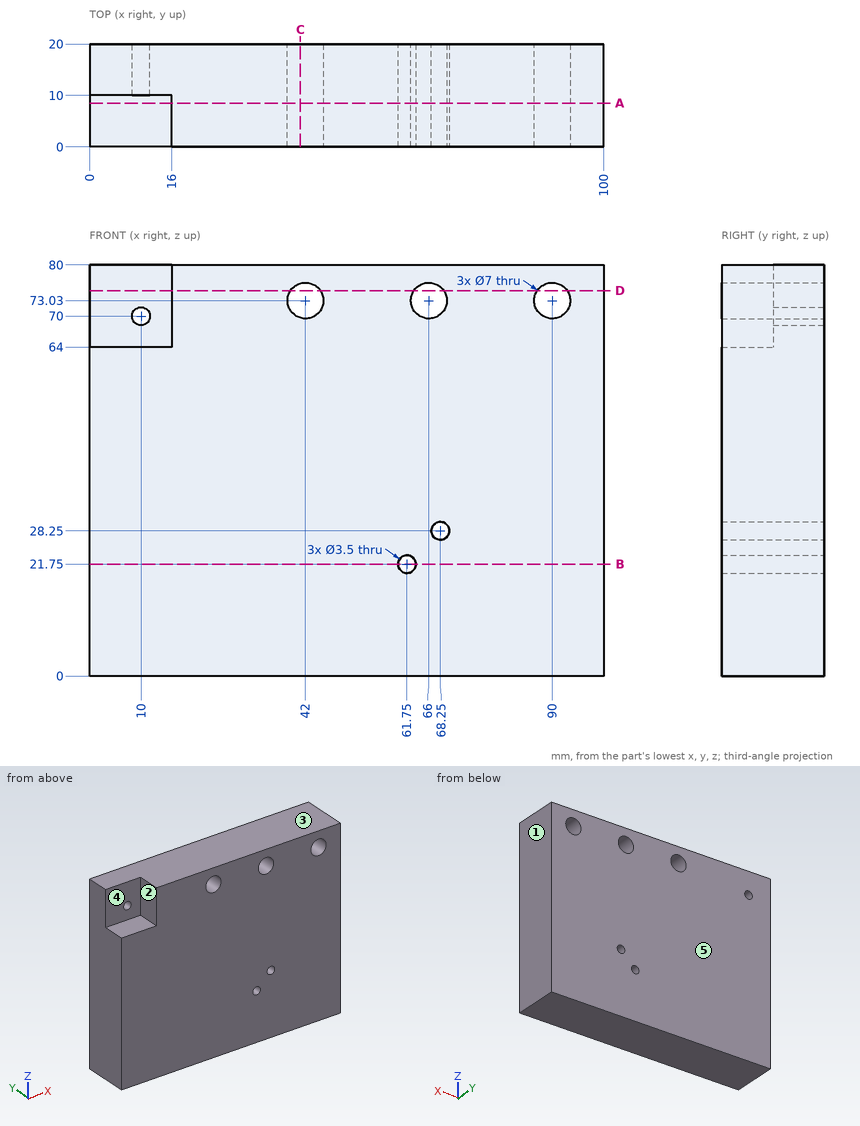
Input: dimensioned drawing with shaded views. Units: mm. Origin: part minimum x, y, z. A direction names the side the tool comes from. Give positions to 0.01 mm unless a question says otherwise; leave off trailing zeros. Order: outer loops, then holes, each group sorted by start corner. A loop starts at its lowest first (then second) coordinate and runs counter-clockwise, first axis right, second up. Notation, with made-up numbers: (70.25, -24.5) -> (117.25, -24.5) arc R14 cw to (117.25, -14.5) -> close; hole circle Ø11 at (85, 43). An arc over 180 degrees is marked (long way). Write item = value, one per line.
Item 1: Ray query, probe 1 along Z at (x, y) = (66, 14); probe 2 along X at (y, z) = (16.5, 70); probe 3 along X at (y, z) = (9.5, 74). Return the intervals inside material, ascending.
Check result:
probe_1 = 0 to 69.53, 76.53 to 80
probe_2 = 0 to 8.25, 11.75 to 40.25, 43.75 to 64.25, 67.75 to 88.25, 91.75 to 100
probe_3 = 16 to 38.64, 45.36 to 62.64, 69.36 to 86.64, 93.36 to 100
Item 2: Contact query for flat-ended pins moving along their axis: pin 1 (4 mm diameter, centred on x = 66, z = 73.03, fed in from -Y); pin 2 (5 mm diameter, centred on x = 9, y = 3, fed in from +Z). Output: stop coordinate, or through.
Check result:
pin_1 = through
pin_2 = 64
Item 3: Section query D-D (z = 75). Output: boundary loops of the cut face in (x, y), then the cut area to 3 significant figures.
Check result:
outline = (0, 10) -> (16, 10) -> (16, 0) -> (39.11, 0) -> (39.11, 20) -> (0, 20) -> close; (44.89, 0) -> (63.11, 0) -> (63.11, 20) -> (44.89, 20) -> close; (68.89, 0) -> (87.11, 0) -> (87.11, 20) -> (68.89, 20) -> close; (92.89, 0) -> (100, 0) -> (100, 20) -> (92.89, 20) -> close
area = 1,490 mm²
Item 4: Section query B-B (z = 21.75). Output: boundary loops of the cut face in (x, y), then the cut area to 3 significant figures.
Check result:
outline = (0, 0) -> (60, 0) -> (60, 20) -> (0, 20) -> close; (63.5, 0) -> (100, 0) -> (100, 20) -> (63.5, 20) -> close
area = 1,930 mm²
Item 5: Mould query, pull axis X, two halves, no side actions, for the marked faces 1, 2 and 3. Classes: +X half, -X half, draft (parallel to the pull), parting line (faces both ways), or undercut.
Check result:
face_1 = +X half
face_2 = -X half
face_3 = draft
Item 6: Section query A-A (y = 8.5). Output: boundary loops of the cut face in (x, z), then the cut area to 3 significant figures.
Check result:
outline = (0, 0) -> (100, 0) -> (100, 80) -> (16, 80) -> (16, 64) -> (0, 64) -> close; hole circle Ø7 at (42, 73.03); hole circle Ø3.5 at (61.75, 21.75); hole circle Ø7 at (66, 73.03); hole circle Ø3.5 at (68.25, 28.25); hole circle Ø7 at (90, 73.03)
area = 7,610 mm²
Item 7: Section query C-C (x = 41). Output: boundary loops of the cut face in (y, z).
Check result:
outline = (0, 0) -> (20, 0) -> (20, 69.68) -> (0, 69.68) -> close; (0, 76.38) -> (20, 76.38) -> (20, 80) -> (0, 80) -> close
Item 8: Set-up query: the marked faces 4 and 5. Return all of +Z, -Z, +X, -X, +Y, -Y with unobstructed straight access to the full face (end or side cutting, diameter ignored); none if empty.
Check result:
face_4 = +Z, -X, -Y
face_5 = +Z, -Z, +X, -X, +Y
